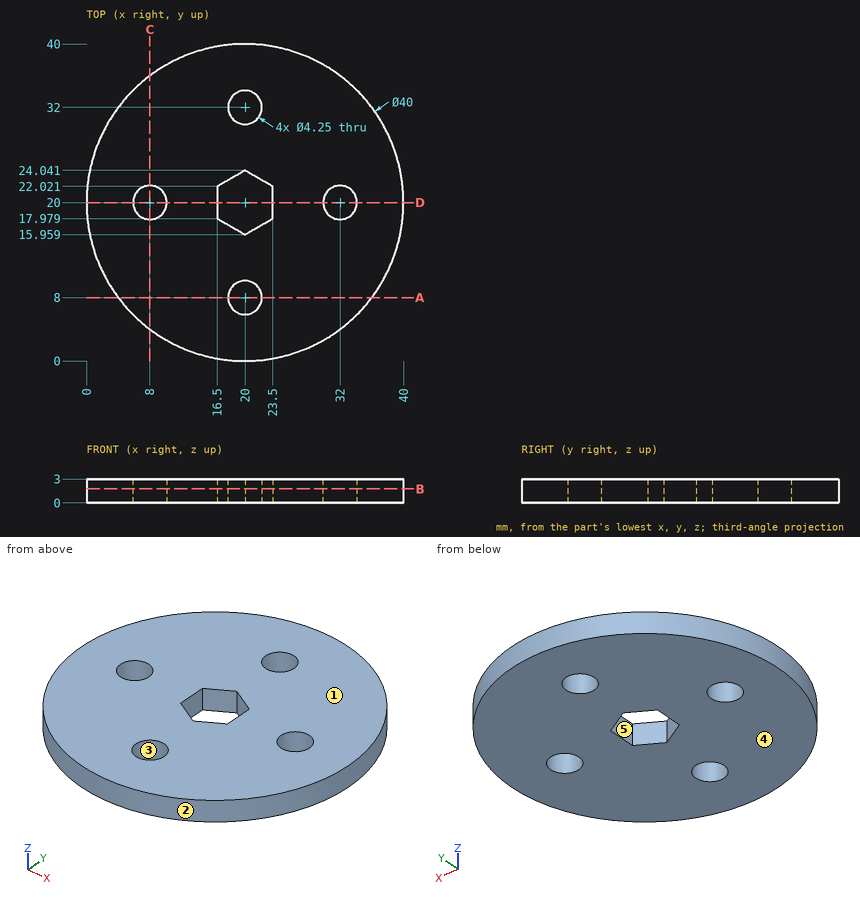
Here's the drawing with two shaded views (mm, measured from the low corner). I have some questions. A direction names the side the tool comes from. Coordinates: 2 decimals unless noted, no trailing zeros. Loops run counter-clockwise (first coordinate to the right, second up) from the corner with the lowest first, then second, coordinate; pieces in that order, holes last. Notation, with made-up numbers: (-15, 48) -> (27, 48) arc R16 ccw to (27, 77) -> close; hole circle Ø5 at (3.25, -10.5). An arc over 180 degrees is marked (long way). Answer as a JSON object with one key per item and string values.
1) For P1, Ø2.5, axis at x = 20, y = 8, coming from the +Z side; P2, Ø1.5, axis at x = 6.5, z = 2.5, coming from the +Y side; P3, Ø1.5, axis at y = 19, z = 1.5, coming from the +X side, each with a flat end and sliding along its axis, tell me the tip position at first contact or that it passes through.
Results:
{"P1": "passes through", "P2": "stops at y = 35.41", "P3": "stops at x = 40"}
2) If I drill on line 1 (Y direction, x = 20, z = 1.5) (1 decimal); line 2 (Y direction, x = 19.5, z = 1.6) (1 decimal); line 3 (Y direction, x = 8, z = 1.75) (1 decimal), over which ranges is the centre line in solid material (lowest first)?
Results:
{"line 1": "y = 0 to 5.9, 10.1 to 16, 24 to 29.9, 34.1 to 40", "line 2": "y = 0 to 5.9, 10.1 to 16.2, 23.8 to 29.9, 34.1 to 40", "line 3": "y = 4 to 17.9, 22.1 to 36"}
3) Imagine slicing it at A-A (y = 8). Please give me the cut outline in (x, z) (1 decimal).
Results:
{"outline": "(4, 0) -> (17.9, 0) -> (17.9, 3) -> (4, 3) -> close; (22.1, 0) -> (36, 0) -> (36, 3) -> (22.1, 3) -> close"}
4) Imagine slicing it at B-B (z = 1.75). Count the separate pieces of the cut face and the enclosed holes in it, then the cut area to 3 significant figures.
Results:
{"separate pieces": "1", "enclosed holes": "5", "area": "1,160 mm^2"}
5) Thinking about a two-plate mould opening in X: for the marked faces 1, 2 and 3, which applies, pulls with the +X half, pulls with the -X half, needs draft (parallel to the pull), parting line crosses it, or undercut?
Results:
{"face 1": "needs draft", "face 2": "parting line crosses it", "face 3": "undercut"}
6) For the marked faces 4 and 5, which set-ups out of +Z, -Z, +X, -X, +Y, -Y let a thin tool reach every point of the face, with its end or its side?
Results:
{"face 4": "-Z, +X, -X, +Y, -Y", "face 5": "+Z, -Z"}
7) Imagine slicing it at D-D (y = 20). Please give me the cut outline in (x, z) (1 decimal).
Results:
{"outline": "(0, 0) -> (5.9, 0) -> (5.9, 3) -> (0, 3) -> close; (10.1, 0) -> (16.5, 0) -> (16.5, 3) -> (10.1, 3) -> close; (23.5, 0) -> (29.9, 0) -> (29.9, 3) -> (23.5, 3) -> close; (34.1, 0) -> (40, 0) -> (40, 3) -> (34.1, 3) -> close"}
